Could you check a few things on this model? Use its own coordinates, in mm. A direction names the side the tool comes from. Coordinates: 2 decimals unless noted, no trailing zeros. Loops run counter-clockwise (first coordinate to the right, second up) from the corner with the lowest first, then second, coordinate; pieces in that order, holes last.
from build123d import *

# Parameters (mm, degrees)
F0_R     = 6.35
F1_DEPTH = 12.7
F2_R     = 6.35
F3_DEPTH = 44.45
F4_SIZE  = 6.35
F5_SIZE  = 6.35
F6_SIZE  = 6.35
F7_SIZE  = 6.35


# Not quite as in the source:
# - a feature names something its author has since deleted; it is built from what else it names


with BuildPart() as f1:
    # F0 (on Front) → F1 (new body, symmetric)
    with BuildSketch(Plane.XZ):
        with BuildLine():
            Line((-14.7091181397, 12.7), (-78.2091181397, 12.7))
            Line((-78.2091181397, 12.7), (-78.2091181397, -12.7))
            Line((-78.2091181397, -12.7), (-14.7091181397, -12.7))
            ThreePointArc((-14.7091181397, -12.7), (-5.7288620187, -16.4197438789), (-2.0091181397, -25.4))
            Line((-2.0091181397, -25.4), (-2.0091181397, -25.5123577416))
            ThreePointArc((-2.0091181397, -25.5123577416), (1.7106257392, -34.4926138626), (10.6908818603, -38.2123577416))
            Line((10.6908818603, -38.2123577416), (99.5908818603, -38.2123577416))
            Line((99.5908818603, -38.2123577416), (99.5908818603, -12.8123577416))
            Line((99.5908818603, -12.8123577416), (36.0908818603, -12.8123577416))
            ThreePointArc((36.0908818603, -12.8123577416), (27.1106257392, -9.0926138626), (23.3908818603, -0.1123577416))
            ThreePointArc((23.3908818603, -0.1123577416), (27.1106257392, 8.8678983795), (36.0908818603, 12.5876422584))
            Line((36.0908818603, 12.5876422584), (99.5908818603, 12.5876422584))
            Line((99.5908818603, 12.5876422584), (99.5908818603, 37.9876422584))
            Line((99.5908818603, 37.9876422584), (10.6908818603, 37.9876422584))
            ThreePointArc((10.6908818603, 37.9876422584), (1.7106257392, 34.2678983795), (-2.0091181397, 25.2876422584))
            Line((-2.0091181397, 25.2876422584), (-2.0091181397, 25.4))
            ThreePointArc((-2.0091181397, 25.4), (-5.7288620187, 16.4197438789), (-14.7091181397, 12.7))
        make_face()
        with Locations((-65.5091181397, 0)):
            Circle(F0_R, mode=Mode.SUBTRACT)
    extrude(amount=F1_DEPTH, both=True)

    # F2 (on Top) → F3 (cut, symmetric)
    with BuildSketch(Plane.XY):
        with Locations((86.8908818603, 0)):
            Circle(F2_R)
    extrude(amount=F3_DEPTH, both=True, mode=Mode.SUBTRACT)

    # F4
    f4_edges = [f1.edges().sort_by_distance(p)[0] for p in [
        (99.590882, -12.7, 25.287642),
    ]]
    chamfer(f4_edges, length=F4_SIZE)

    # F5
    f5_edges = [f1.edges().sort_by_distance(p)[0] for p in [
        (99.590882, 12.7, 25.287642),
    ]]
    chamfer(f5_edges, length=F5_SIZE)

    # F6
    f6_edges = [f1.edges().sort_by_distance(p)[0] for p in [
        (99.590882, -12.7, -25.512358),
    ]]
    chamfer(f6_edges, length=F6_SIZE)

    # F7
    f7_edges = [f1.edges().sort_by_distance(p)[0] for p in [
        (99.590882, 12.7, -25.512358),
    ]]
    chamfer(f7_edges, length=F7_SIZE)


solid = f1.part
1) Imagine slicing it at D-D on y = 9.75. List the corners of the cut face in (x, z) for me, plus the area to 3 significant figures.
2) Imagine slicing it at B-B on y = 0. List the corners of the cut face in (x, z) for me.
3) Imagine slicing it at C-C on z = 17.5. List the corners of the cut face in (x, y) for me.
4) For faces 5 (the flat face through (-46, 0, 12.7)), 6 (the flat face through (68, 0, -12.812)), 7 (the cylindrical face through (-71.853, 0.178, 0.279)), which set-ups out of +Z, -Z, +X, -X, +Y, -Y let a thin tool reach every point of the face, with its end or its side?
5) We'd pull the mould along Y, two halves only. Please class faces 1 (the cylindrical face through (92.948, 1.907, 25.465)), 2 (the flat face through (67, 0, 12.588)), 3 (the flat face through (25, -12.7, 9)), 4 (the flat face through (96.37, 9.57, 25.11)): released by +Y, released by -Y, zero draft, split by the parting line, or undercut.
6) Imagine slicing it at A-A on x = 70.5. List the corners of the cut face in (y, z) for me, plus the area to 3 significant figures.
7) Will these pins go through, and if not, where does the flat tip stop? pin 1 (11.5 mm diameter, centred on x = 86.89, y = 0, fed in from -Z); pin 2 (2 mm diameter, centred on y = -9.5, z = -23, fed in from +X); pin 3 (7.5 mm diameter, centred on x = -48, y = 0.5, fed in from -Z); pin 4 (10 mm diameter, centred on x = -48, y = -6.5, fed in from +Z).
8) If I drill on L1, parallel to Z at x = 62, y = -6; L2, parallel to Y at x = 85.5, z = -30.5; L3, parallel to Y at x = 87, z = 17, over which ranges is the centre line in solid material (lowest first)?
Solved:
1. outline: (-78.21, -12.7) - (-14.71, -12.7) arc R12.7 cw to (-2.01, -25.4) - (-2.01, -25.51) arc R12.7 ccw to (10.69, -38.21) - (96.19, -38.21) - (96.19, -12.81) - (36.09, -12.81) arc R12.7 cw to (36.09, 12.59) - (96.19, 12.59) - (96.19, 37.99) - (10.69, 37.99) arc R12.7 ccw to (-2.01, 25.29) - (-2.01, 25.4) arc R12.7 cw to (-14.71, 12.7) - (-78.21, 12.7) - close; hole circle Ø12.7 at (-65.51, 0)
1. area: 7,510 mm2
2. outline: (-78.21, -12.7) - (-14.71, -12.7) arc R12.7 cw to (-2.01, -25.4) - (-2.01, -25.51) arc R12.7 ccw to (10.69, -38.21) - (80.54, -38.21) - (80.54, -12.81) - (36.09, -12.81) arc R12.7 cw to (36.09, 12.59) - (80.54, 12.59) - (80.54, 37.99) - (10.69, 37.99) arc R12.7 ccw to (-2.01, 25.29) - (-2.01, 25.4) arc R12.7 cw to (-14.71, 12.7) - (-78.21, 12.7) - close; (93.24, -38.21) - (99.59, -38.21) - (99.59, -12.81) - (93.24, -12.81) - close; (93.24, 12.59) - (99.59, 12.59) - (99.59, 37.99) - (93.24, 37.99) - close; hole circle Ø12.7 at (-65.51, 0)
3. outline: (-4.77, -12.7) - (93.24, -12.7) - (99.59, -6.35) - (99.59, 6.35) - (93.24, 12.7) - (-4.77, 12.7) - close; hole circle Ø12.7 at (86.89, 0)
4. face 5: +Z, -X, +Y, -Y
4. face 6: +X, +Y, -Y
4. face 7: +Y, -Y
5. face 1: undercut
5. face 2: zero draft
5. face 3: released by -Y
5. face 4: released by +Y
6. outline: (-12.7, -38.21) - (12.7, -38.21) - (12.7, -12.81) - (-12.7, -12.81) - close; (-12.7, 12.59) - (12.7, 12.59) - (12.7, 37.99) - (-12.7, 37.99) - close
6. area: 1,290 mm2
7. pin 1: passes through
7. pin 2: stops at x = 97.44
7. pin 3: stops at z = -12.7
7. pin 4: stops at z = 12.7
8. L1: z = -38.21 to -12.81, 12.59 to 37.99
8. L2: y = -12.7 to -6.2, 6.2 to 12.7
8. L3: y = -12.7 to -6.35, 6.35 to 12.7
